Source: three-view drawing plus pictorial views. Frame: mm from the lowest corner of the part. A direction names the side the tool comes from. Give positions to 0.01 mm unless a question says otherwise; leave off trailing zeros. Loops run counter-clockwise (first coordinate to the right, second up) from the corner with the lowest first, then second, coordinate; pieces in that order, holes last. Notation, with made-up numbers: M -32.75,14 L -26.75,14 A13 cw -26.75,29 Z; hole C 60.5,50.5 d9. An arc over 180 degrees is marked long. One line per item, written item: value. Start each with the question number.
(1) Pull-direction query (Y, two-part tool) for the marked faces 4, 5 and 6; classes: released by +Y, released by -Y, zero draft, split by the parting line, or undercut.
(2) Pin query (flat end, axial travel): P1, Ø3, axis at y = 32, z = 22, coming from the +X side; P2, Ø11.5, axis at x = 17.5, z = 9, coming from the +Y side; P3, Ø11.5, axis at x = 16, z = 16, coming from the -Y side. Return the tip coordinate at first contact, or that it passes through.
(3) Ray query, line 1 along Y through (x, z) = (15.5, 15.25); line 2 along X through (y, z) = (18, 18.5); line 3 along Z through (x, y) = (9, 36). Return the intervals inside material, ascending. Write a range as from..to.
(4) Section D-D on y = 15. State how many separate pieces and enclosed holes the cut face has.
(5) Section B-B on y = 19.5. Output: boundary loops of the cut face in (x, z).
(6) Section C-C on x = 14. Output: boundary loops of the cut face in (y, z).
(7) Access query for the marked faces 1, 2 and 3. Directions: +Z, -Z, +X, -X, +Y, -Y. A direction counts if a zero-diameter tool reaches every point of the face in a straight line with its end or side. Return the directions, or none.
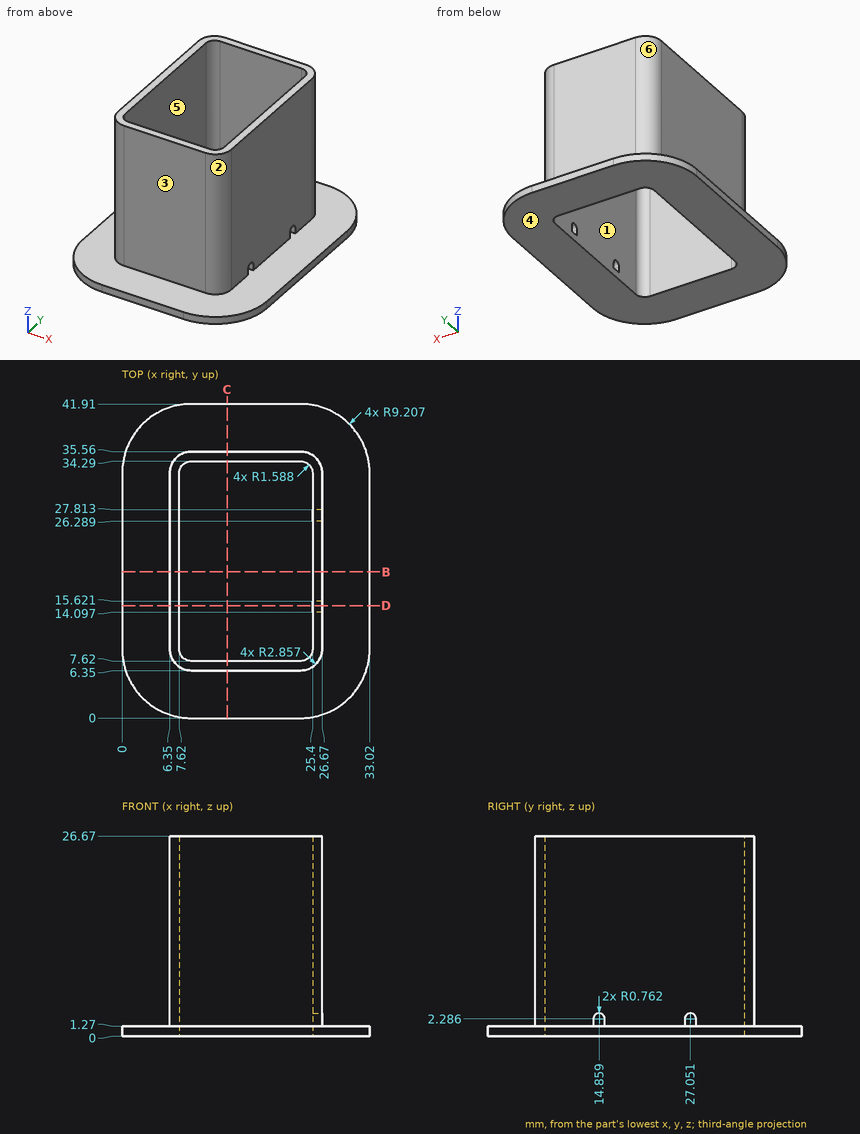
Output values:
1. face 4: zero draft
1. face 5: undercut
1. face 6: released by +Y
2. P1: stops at x = 26.67
2. P2: stops at y = 35.56
2. P3: stops at y = 6.35
3. line 1: y = 6.35..7.62, 34.29..35.56
3. line 2: x = 6.35..7.62, 25.4..26.67
3. line 3: z = 0..1.27
4. separate pieces: 3
4. enclosed holes: 0
5. outline: M 0,0 L 7.62,0 L 7.62,26.67 L 6.35,26.67 L 6.35,1.27 L 0,1.27 Z; M 25.4,0 L 33.02,0 L 33.02,1.27 L 26.67,1.27 L 26.67,26.67 L 25.4,26.67 Z
6. outline: M 0,0 L 7.62,0 L 7.62,26.67 L 6.35,26.67 L 6.35,1.27 L 0,1.27 Z; M 34.29,0 L 41.91,0 L 41.91,1.27 L 35.56,1.27 L 35.56,26.67 L 34.29,26.67 Z
7. face 1: +Z, -Z
7. face 2: +Z, +X, -Y
7. face 3: +Z, +X, -X, -Y
